from build123d import *

# Parameters (mm, degrees)
DODANIE_WYCI_GNI_CIE1_DEPTH    = 77.5
SZKIC2_W                       = 46
SZKIC2_H                       = 50.5
DODANIE_WYCI_GNI_CIE2_DEPTH    = 3
SZKIC3_W                       = 1
SZKIC3_H                       = 50.5
DODANIE_WYCI_GNI_CIE3_DEPTH    = 22
SZKIC4_W                       = 8
SZKIC4_H                       = 50.5
WYTNIJ_WYCI_GNI_CIE1_DEPTH     = 1
SFAZOWANIE1_SIZE               = 1
OTWORY_USTALAJ_CE_5_0MM1_D     = 5
OTWORY_USTALAJ_CE_5_0MM1_DEPTH = 10
OTWORY_USTALAJ_CE_5_0MM1_TIP   = 1.502151548


with BuildPart() as part:
    # Szkic1 → Dodanie-wyciągnięcie1 (new body)
    with BuildSketch(Plane.XY):
        Polygon((-10, 0), (-10, 4), (-6, 8), (-6, 10), (-10, 14), (-10, 15), (-7.5, 17.5), (7.5, 17.5), (10, 15), (10, 14), (6, 10), (6, 8), (10, 4), (10, 0), (22, 0), (22, 22), (-22, 22), (-22, 0), align=None)
    extrude(amount=DODANIE_WYCI_GNI_CIE1_DEPTH)

    # Szkic2 → Dodanie-wyciągnięcie2 (add)
    with BuildSketch(Plane(origin=(0, 22, 0), x_dir=(1, 0, 0), z_dir=(0, 1, 0))):
        with Locations((0, -38.75)):
            Rectangle(SZKIC2_W, SZKIC2_H)
    extrude(amount=DODANIE_WYCI_GNI_CIE2_DEPTH)

    # Szkic3 → Dodanie-wyciągnięcie3 (add)
    with BuildSketch(Plane.XZ.offset(-22)):
        with Locations((-22.5, 38.75)):
            Rectangle(SZKIC3_W, SZKIC3_H)
        with Locations((22.5, 38.75)):
            Rectangle(SZKIC3_W, SZKIC3_H)
    extrude(amount=DODANIE_WYCI_GNI_CIE3_DEPTH)

    # Szkic4 → Wytnij-wyciągnięcie1 (cut)
    with BuildSketch(Plane(origin=(0, 25, 0), x_dir=(1, 0, 0), z_dir=(0, 1, 0))):
        with Locations((-9, -38.75)):
            Rectangle(SZKIC4_W, SZKIC4_H)
        with Locations((9, -38.75)):
            Rectangle(SZKIC4_W, SZKIC4_H)
    extrude(amount=-WYTNIJ_WYCI_GNI_CIE1_DEPTH, mode=Mode.SUBTRACT)

    # Sfazowanie1
    sfazowanie1_edges = [part.edges().sort_by_distance(p)[0] for p in [
        (-23, 25, 38.75),
        (-13, 25, 38.75),
        (-5, 25, 38.75),
        (5, 25, 38.75),
        (13, 25, 38.75),
        (23, 25, 38.75),
    ]]
    chamfer(sfazowanie1_edges, length=SFAZOWANIE1_SIZE - 0.0001)  # a hair under: the kernel refuses the full size

    # Otwory ustalające Ø5.0mm1
    with Locations(Plane(origin=(0, 25, 0), x_dir=(1, 0, 0), z_dir=(0, 1, 0))):
        with Locations((-18, -20.75), (18, -20.75), (18, -56.75), (-18, -56.75)):
            Hole(OTWORY_USTALAJ_CE_5_0MM1_D / 2, depth=OTWORY_USTALAJ_CE_5_0MM1_DEPTH)
            with Locations((0, 0, -(OTWORY_USTALAJ_CE_5_0MM1_DEPTH + OTWORY_USTALAJ_CE_5_0MM1_TIP / 2))):  # 118° drill point
                Cone(0, OTWORY_USTALAJ_CE_5_0MM1_D / 2, OTWORY_USTALAJ_CE_5_0MM1_TIP, mode=Mode.SUBTRACT)


solid = part.part
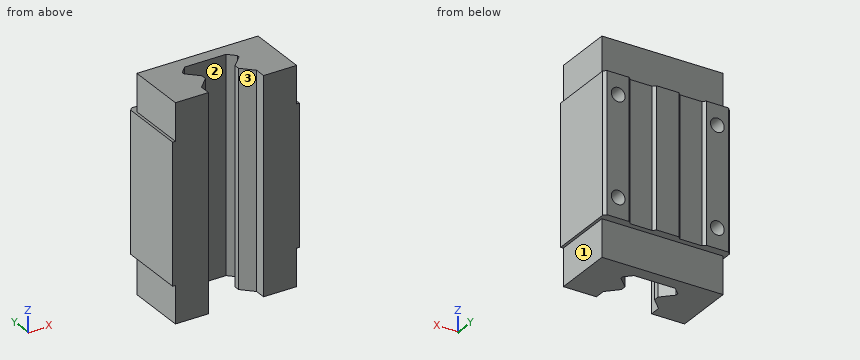
Build history of the part. All positions in model axes, mm. Face numbers are marked on the shaded views. A direction names the side the tool comes from. Coordinates: 2 decimals unless noted, no trailing zeros. Order: outer loops, then holes, each group sorted by start corner. A loop starts at its lowest first (then second) coordinate and runs counter-clockwise, first axis right, second up. Notation, with made-up numbers: (41.25, 8.25) - (59.25, 8.25) arc R22 ccw to (59.25, 18.25) - close; hole circle Ø1 at (-2, 62). An arc over 180 degrees is marked (long way). Write item = value, one per line. Start each with the question number.
1) Flat gauge pins, fed straight in: pin 1 Ø4.5 at (x, z) = (-18, 56.75) entering from +Y; pin 2 Ø15 at (y, z) = (11, 69.5) entering from +X; pin 3 Ø7 at (y, z) = (14, 4) entering from -X; pin 4 Ø12 at (x, z) = (1.5, 47.5) entering from -Y. Where does each tip first touch, or does it go through?
2) Saw through at B-B on y = 16.5. Write the cut outline in (x, z).
3) Saw through at A-A on y = 6.5. Write the cut outline in (x, z), then the cut area to 3 significant figures.
4) Wall check: line 1 along Z through (x, y) = (-18, 23.25); line 2 along X through (y, z) = (20.25, 56.75); line 3 along Z through (x, y) = (-18, 20.5). Give the ranges that are in metal, low to high. Write a range as from..to.
5) 3-axis set-ups, long thin cutter, end or side, ignore diameter. For the marked faces 1, 2 and 3: which of +Z, -Z, +X, -X, +Y, -Y reach the whole face in a straight line?
6) Saw through at D-D on y = 20.5. Write the cut outline in (x, z).
From the geometry:
q1.pin_1 = 14.85
q1.pin_2 = 23
q1.pin_3 = -22
q1.pin_4 = 6.5
q2.outline = (-23, 13.5) - (-22, 13.5) - (-22, 0) - (-8.5, 0) - (-8.5, 77.5) - (-22, 77.5) - (-22, 64) - (-23, 64) - close; (8.5, 0) - (22, 0) - (22, 13.5) - (23, 13.5) - (23, 64) - (22, 64) - (22, 77.5) - (8.5, 77.5) - close; hole circle Ø5 at (-18, 20.75); hole circle Ø5 at (-18, 56.75); hole circle Ø5 at (18, 20.75); hole circle Ø5 at (18, 56.75)
q3.outline = (-23, 13.5) - (-22, 13.5) - (-22, 0) - (-7.5, 0) - (-7.5, 77.5) - (-22, 77.5) - (-22, 64) - (-23, 64) - close; (7.5, 0) - (22, 0) - (22, 13.5) - (23, 13.5) - (23, 64) - (22, 64) - (22, 77.5) - (7.5, 77.5) - close
q3.area = 2,350 mm^2
q4.line_1 = 13.5..18.25, 23.25..54.25, 59.25..64
q4.line_2 = -23..-20.5, -15.5..15.5, 20.5..23
q4.line_3 = 0..18.25, 23.25..54.25, 59.25..77.5
q5.face_1 = -Z, +X, +Y, -Y
q5.face_2 = +Z, -Z
q5.face_3 = +Z, -Z, -Y
q6.outline = (-23, 13.5) - (-22, 13.5) - (-22, 0) - (22, 0) - (22, 13.5) - (23, 13.5) - (23, 64) - (22, 64) - (22, 77.5) - (-22, 77.5) - (-22, 64) - (-23, 64) - close; hole circle Ø5 at (-18, 20.75); hole circle Ø5 at (-18, 56.75); hole circle Ø5 at (18, 20.75); hole circle Ø5 at (18, 56.75)
